```python
from build123d import *

# Parameters (mm, degrees)
SKETCH_1_R          = 16.075
SKETCH_1_R_2        = 12.575
EXTRUDE_1_DEPTH     = 7.5
SKETCH_2_R          = 16.075
EXTRUDE_2_DEPTH     = 2
SKETCH_3_R          = 20
EXTRUDE_3_DEPTH     = 6
FILLET_1_R          = 5
CUT_EXTRUDE_1_DEPTH = 1
EXTRUDE_4_DEPTH     = 7
CUT_EXTRUDE_2_DEPTH = 4.5
FILLET_2_R          = 3
FILLET_3_R          = 10
FILLET_4_R          = 1


with BuildPart() as part:
    # 草图1 → 凸台-拉伸1 (new body)
    with BuildSketch(Plane.XY):
        Circle(SKETCH_1_R)
        Circle(SKETCH_1_R_2, mode=Mode.SUBTRACT)
    extrude(amount=EXTRUDE_1_DEPTH)

    # 草图2 → 凸台-拉伸2 (add)
    with BuildSketch(Plane.XY.offset(7.5)):
        Circle(SKETCH_2_R)
    extrude(amount=EXTRUDE_2_DEPTH)

    # 草图3 → 凸台-拉伸3 (add)
    with BuildSketch(Plane.XY.offset(9.5)):
        Circle(SKETCH_3_R)
    extrude(amount=EXTRUDE_3_DEPTH)

    # 圆角1
    fillet_1_edges = [part.edges().sort_by_distance(p)[0] for p in [
        (-20, 0, 15.5),
    ]]
    fillet(fillet_1_edges, radius=FILLET_1_R)

    # 草图4 → 切除-拉伸1 (cut)
    with BuildSketch(Plane.XY.offset(15.5)):
        with BuildLine():
            Line((9.757359313, 1.242640687), (0, 11))
            Line((0, 11), (-9.757359313, 1.242640687))
            ThreePointArc((-9.757359313, 1.242640687), (-8.878650761, -7.968295542), (0, -5.363869387))
            ThreePointArc((0, -5.363869387), (8.878650761, -7.968295542), (9.757359313, 1.242640687))
        make_face()
    extrude(amount=-CUT_EXTRUDE_1_DEPTH, mode=Mode.SUBTRACT)

    # 草图6 → 凸台-拉伸4 (add, symmetric)
    with BuildSketch(Plane(origin=(0, 0, 0), x_dir=(1, 0, 0), z_dir=(0, 1, 0))):
        Polygon((10.75, -5), (11.05, 0), (14, 0), (14, -7.5), (10.6, -7.5), align=None)
    extrude_4 = extrude(amount=EXTRUDE_4_DEPTH, both=True)

    # 镜向1: 凸台-拉伸4 across plane
    add(extrude_4.mirror(Plane(origin=(0, 0, 0), x_dir=(0, 0, 1), z_dir=(1, 0, 0))))

    # 草图5 → 切除-拉伸2 (cut)
    with BuildSketch(Plane(origin=(0, 0, 7.5), x_dir=(-1, 0, 0), z_dir=(0, 0, -1))):
        with BuildLine():
            Line((7.767720909, 9.889041252), (0, 2.121320344))
            Line((0, 2.121320344), (-7.767720909, 9.889041252))
            ThreePointArc((-7.767720909, 9.889041252), (0, 12.575), (7.767720909, 9.889041252))
        make_face()
        with BuildLine():
            Line((-7.767720909, -9.889041252), (0, -2.121320344))
            Line((0, -2.121320344), (7.767720909, -9.889041252))
            ThreePointArc((7.767720909, -9.889041252), (0, -12.575), (-7.767720909, -9.889041252))
        make_face()
        with BuildLine():
            Line((-9.889041252, 7.767720909), (-2.121320344, 0))
            Line((-2.121320344, 0), (-9.889041252, -7.767720909))
            ThreePointArc((-9.889041252, -7.767720909), (-10.256771671, -7.275249816), (-10.6, -6.765399101))
            Line((-10.6, -6.765399101), (-10.6, 6.765399101))
            ThreePointArc((-10.6, 6.765399101), (-10.256771671, 7.275249816), (-9.889041252, 7.767720909))
        make_face()
        with BuildLine():
            Line((2.121320344, 0), (9.889041252, 7.767720909))
            ThreePointArc((9.889041252, 7.767720909), (10.256771671, 7.275249816), (10.6, 6.765399101))
            Line((10.6, 6.765399101), (10.6, -6.765399101))
            ThreePointArc((10.6, -6.765399101), (10.256771671, -7.275249816), (9.889041252, -7.767720909))
            Line((9.889041252, -7.767720909), (2.121320344, 0))
        make_face()
    extrude(amount=-CUT_EXTRUDE_2_DEPTH, mode=Mode.SUBTRACT)

    # 圆角2
    fillet_2_edges = [part.edges().sort_by_distance(p)[0] for p in [
        (-16.075, 0, 9.5),
    ]]
    fillet(fillet_2_edges, radius=FILLET_2_R)

    # 圆角3
    # the kernel refuses this fillet: 10 mm, written as the material it takes off along each edge
    with BuildSketch(Plane(origin=(10.6, -7.514725314, 7.5), x_dir=(0.05989229072795002, 0, -0.9982048454657784), z_dir=(0, 1, 0))) as fillet_3_piece_1_section:
        with BuildLine():
            CenterArc((FILLET_3_R * 0.0299730484909, -FILLET_3_R), FILLET_3_R, 90, 3.433630362)
            Line((-FILLET_3_R * 0.029919242237, -FILLET_3_R * 0.00179515453422), (0, 0))
            Line((0, 0), (FILLET_3_R * 0.0299730484909, 0))
        make_face()
    fillet_3_piece_1 = extrude(amount=15.029450627, mode=Mode.PRIVATE)
    fillet_3_piece_1 = fillet_3_piece_1 & Plane(origin=(0, 0, 7.497328359), x_dir=(1, 0, 0), z_dir=(0, 0, -1)) * Cylinder(12.575, 32, mode=Mode.PRIVATE)
    add(fillet_3_piece_1, mode=Mode.SUBTRACT)
    with BuildSketch(Plane(origin=(-10.6, -7.514725314, 7.5), x_dir=(-0.05989229072795002, 0, -0.9982048454657784), z_dir=(0, 1, 0))) as fillet_3_piece_2_section:
        with BuildLine():
            CenterArc((FILLET_3_R * 0.0299730484909, FILLET_3_R), FILLET_3_R, 266.566369638, 3.433630362)
            Line((-FILLET_3_R * 0.029919242237, FILLET_3_R * 0.00179515453422), (0, 0))
            Line((0, 0), (FILLET_3_R * 0.0299730484909, 0))
        make_face()
    fillet_3_piece_2 = extrude(amount=15.029450627, mode=Mode.PRIVATE)
    fillet_3_piece_2 = fillet_3_piece_2 & Plane(origin=(0, 0, 7.497328359), x_dir=(1, 0, 0), z_dir=(0, 0, -1)) * Cylinder(12.575, 32, mode=Mode.PRIVATE)
    add(fillet_3_piece_2, mode=Mode.SUBTRACT)

    # 圆角4
    # the kernel refuses this fillet: 1 mm, written as the material it adds along each edge
    with BuildSketch(Plane(origin=(0, -2.121320344, 7.5), x_dir=(0.7071067811865518, -0.7071067811865432, 0), z_dir=(0, 0, 1)), Plane(origin=(2.121320344, 0, 7.5), x_dir=(0.7071067811865438, 0.7071067811865512, 0), z_dir=(0, 0, 1))) as fillet_4_piece_1:
        with BuildLine():
            CenterArc((FILLET_4_R, -FILLET_4_R), FILLET_4_R, 90, 90)
            Line((0, -FILLET_4_R), (0, 0))
            Line((0, 0), (FILLET_4_R, 0))
        make_face()
    extrude(amount=7)
    with BuildSketch(Plane(origin=(-7.767720909, -9.889041252, 7.5), x_dir=(0.8157540941110909, -0.5783988744292242, 0), z_dir=(0, 0, 1)), Plane(origin=(-9.889041252, 7.767720909, 7.5), x_dir=(-0.5783988744292212, -0.8157540941110929, 0), z_dir=(0, 0, 1)), Plane(origin=(7.767720909, 9.889041252, 7.5), x_dir=(-0.8157540941110928, 0.5783988744292216, 0), z_dir=(0, 0, 1))) as fillet_4_piece_2:
        with BuildLine():
            CenterArc((1.184434693, 0.998796574), FILLET_4_R, 170.338006618, 102.473187785)
            Line((0.198619674, 1.166632059), (0, 0))
            ThreePointArc((0, 0), (0.616739804, -0.015133081), (1.233479607, 0))
        make_face()
    extrude(amount=7.583699018)
    with BuildSketch(Plane(origin=(-9.889041252, -7.767720909, 7.5), x_dir=(-0.578398874429234, 0.8157540941110841, 0), z_dir=(0, 0, 1))) as fillet_4_piece_3_section:
        with BuildLine():
            CenterArc((1.184434693, -0.998796574), FILLET_4_R, 87.188805597, 102.473187785)
            Line((0.198619674, -1.166632059), (0, 0))
            ThreePointArc((0, 0), (0.616739804, 0.015133081), (1.233479607, 0))
        make_face()
    fillet_4_piece_3 = extrude(amount=7.583699018, mode=Mode.PRIVATE)
    fillet_4_piece_3 = split(fillet_4_piece_3, bisect_by=Plane(origin=(-10.600515055, -6.764586018, 14.5), z_dir=(0, 0, -1)), keep=Keep.TOP, mode=Mode.PRIVATE)
    add(fillet_4_piece_3)
    with BuildSketch(Plane(origin=(-2.121320344, 0, 7.5), x_dir=(-0.7071067811865511, 0.7071067811865441, 0), z_dir=(0, 0, 1)), Plane(origin=(0, 2.121320344, 7.5), x_dir=(0.7071067811865439, 0.7071067811865512, 0), z_dir=(0, 0, 1))) as fillet_4_piece_4:
        with BuildLine():
            CenterArc((FILLET_4_R, FILLET_4_R), FILLET_4_R, 180, 90)
            Line((0, FILLET_4_R), (0, 0))
            Line((0, 0), (FILLET_4_R, 0))
        make_face()
    extrude(amount=7)
    with BuildSketch(Plane(origin=(-7.767720909, 9.889041252, 7.5), x_dir=(0.8157540941110883, 0.5783988744292278, 0), z_dir=(0, 0, 1)), Plane(origin=(9.889041252, 7.767720909, 7.5), x_dir=(0.5783988744292311, -0.8157540941110861, 0), z_dir=(0, 0, 1)), Plane(origin=(7.767720909, -9.889041252, 7.5), x_dir=(-0.8157540941110859, -0.5783988744292314, 0), z_dir=(0, 0, 1))) as fillet_4_piece_5:
        with BuildLine():
            CenterArc((1.184434693, -0.998796574), FILLET_4_R, 87.188805597, 102.473187785)
            Line((0.198619674, -1.166632059), (0, 0))
            ThreePointArc((0, 0), (0.616739804, 0.015133081), (1.233479607, 0))
        make_face()
    extrude(amount=7.583699018)
    with BuildSketch(Plane(origin=(9.889041252, -7.767720909, 7.5), x_dir=(0.5783988744292226, 0.8157540941110919, 0), z_dir=(0, 0, 1))) as fillet_4_piece_6_section:
        with BuildLine():
            CenterArc((1.184434693, 0.998796574), FILLET_4_R, 170.338006618, 102.473187785)
            Line((0.198619674, 1.166632059), (0, 0))
            ThreePointArc((0, 0), (0.616739804, -0.015133081), (1.233479607, 0))
        make_face()
    fillet_4_piece_6 = extrude(amount=7.583699018, mode=Mode.PRIVATE)
    fillet_4_piece_6 = split(fillet_4_piece_6, bisect_by=Plane(origin=(10.600515055, -6.764586018, 14.5), z_dir=(0, 0, -1)), keep=Keep.TOP, mode=Mode.PRIVATE)
    add(fillet_4_piece_6)


solid = part.part
```
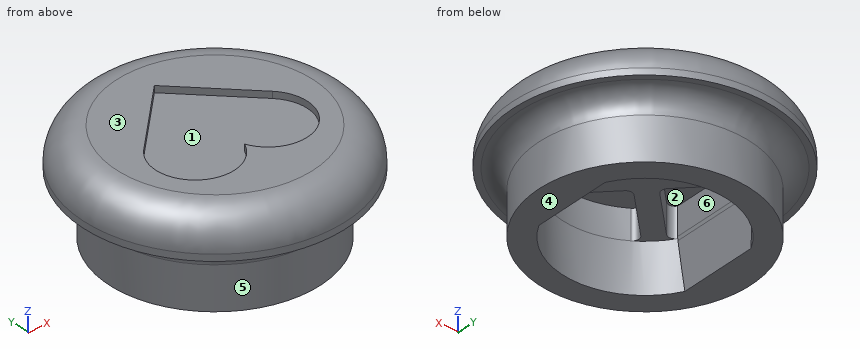
Part model, mm, in its own coordinate system. Face numbers are marked on the shaded views. A direction names the side the tool comes from. Give positions to 0.01 mm unless a question says otherwise; leave off trailing zeros. Order: outer loops, then holes, each group sorted by start corner. A loop starts at its lowest first (then second) coordinate and runs counter-clockwise, first axis right, second up. Notation, with made-up numbers: (13, 56) - (41, 56) arc R32 ccw to (41, 95) - close; hole circle Ø5 at (-22.5, -23.75). An arc over 180 degrees is marked (long way). Use one line per item in the form item = value.
Item 1: Two-plate mould, pull along Y, no slides. Class the marked faces 4, 5 and 6: released by +Y, released by -Y, zero draft, split by the parting line, or undercut.
Solution:
face_4 = zero draft
face_5 = split by the parting line
face_6 = undercut
Item 2: Which spindle directions (+Z, -Z, +X, -X, +Y, -Y) get a long thin tool onto all of the face, cutting with end or side? Do the marked faces 1, 2 and 3. Say none if no direction does.
Solution:
face_1 = +Z
face_2 = -Z
face_3 = +Z, +X, -X, +Y, -Y
Item 3: Probe probe 1 along Y at (x, z) = (-1, 11); probe 2 along Z at (x, y) = (-3, 3.5); probe 3 along Y at (x, z) = (-9, 2.75). List the from-to ranges inside material, lowest first. Write a range as from..to.
Solution:
probe_1 = -19.95..-12.54, -3.12..3.12, 12.54..19.95
probe_2 = 7.5..14.5
probe_3 = -13.32..-8.78, 8.78..13.32
Item 4: Slice it at C-C on z = 1.5. Give the cut face in (x, y) (3 decimals), and give its area (3 significant figures).
Solution:
outline = circle Ø32.15 at (0, 0); hole (-10.96, -6.165) arc R12.575 ccw to (10.96, -6.165) - (10.96, 6.165) arc R12.575 ccw to (-10.96, 6.165) - close
area = 342 mm2
Item 5: Slice it at A-A on z = 5.25. Give the cut face in (x, y) (3 decimals), and give its area (3 significant figures).
Solution:
outline = circle Ø32.15 at (0, 0); hole (-10.735, -6.549) arc R12.575 ccw to (10.735, -6.549) - (10.735, 6.549) arc R12.575 ccw to (-10.735, 6.549) - close
area = 348 mm2
Item 6: Slice it at B-B on y = 0. Give the cut face in (x, z) (3 decimals).
Solution:
outline = (-20, 9.5) - (-19.075, 9.5) arc R3 cw to (-16.075, 6.5) - (-16.075, 0) - (-11.05, 0) - (-10.618, 7.201) arc R10 ccw to (-10.6, 7.8) - (-10.6, 12) - (-2.536, 12) - (-2.536, 7.5) - (2.536, 7.5) - (2.536, 12) - (10.6, 12) - (10.6, 7.8) arc R10 ccw to (10.618, 7.201) - (11.05, 0) - (16.075, 0) - (16.075, 6.5) arc R3 cw to (19.075, 9.5) - (20, 9.5) - (20, 10.5) arc R5 ccw to (15, 15.5) - (10.711, 15.5) - (10.711, 14.5) - (-10.711, 14.5) - (-10.711, 15.5) - (-15, 15.5) arc R5 ccw to (-20, 10.5) - close
Item 7: Pin check, flat tips, straight feed: pin 1 Ø5 at (x, z) = (-5, 5.5) entering from +Y; pin 2 Ø3 at (x, y) = (1, -6.5) entering from -Z; pin 3 Ø6 at (x, z) = (3.5, 3) entering from -Y. Stop position of each tip, or through.
Solution:
pin_1 = 15.88
pin_2 = 12
pin_3 = -16.07
